The listing builds one solid part. Answer for the finished solid, in the listing's coordinates (mm). Coordinates: 2 decimals unless noted, no trailing zeros. Order: outer loops, then holes, each group sorted by start corner. A loop starts at its lowest first (then second) coordinate and runs counter-clockwise, first axis right, second up. Notation, with made-up numbers: (88.25, 59) -> (113.25, 59) arc R24 ccw to (113.25, 78) -> close; hole circle Ø8 at (78, 10.25). An arc over 180 degrees is marked (long way). Return JSON: item names as keys, results as strings.
```python
from build123d import *

# Parameters (mm, degrees)
BOSS_EXTRUDE1_DEPTH       = 10
FILLET2_R                 = 0.5
SKETCH2_R                 = 1.6
CUT_EXTRUDE1_DEPTH        = 4.896527904
REVISION_INDICATION_DEPTH = 0.4


with BuildPart() as part:
    # Sketch1 → Boss-Extrude1 (new body)
    with BuildSketch(Plane(origin=(0, 0, 0), x_dir=(1, 0, 0), z_dir=(0, 1, 0))):
        Polygon((20.35, 0.1), (14.35, 0.1), (0, 0), (-0.016724739, 2.4), (14.35, 3.9), (20.35, 3.9), (34.716724739, 2.4), (34.7, 0), align=None)
    extrude(amount=BOSS_EXTRUDE1_DEPTH)

    # Fillet2
    fillet2_edges = [part.edges().sort_by_distance(p)[0] for p in [
        (-0.016724739, 5, -2.4),
        (34.716724739, 5, -2.4),
        (34.7, 5, 0),
        (0, 5, 0),
    ]]
    fillet(fillet2_edges, radius=FILLET2_R)

    # Sketch2 → Cut-Extrude1 (cut, through all)
    with BuildSketch(Plane(origin=(0, 0, -3.9), x_dir=(-1, 0, 0), z_dir=(0, 0, -1))):
        with Locations((-17.35, 5)):
            Circle(SKETCH2_R)
    extrude(amount=-CUT_EXTRUDE1_DEPTH, mode=Mode.SUBTRACT)

    # Sketch5 → revision indication (add)
    with BuildSketch(Plane(origin=(-0.248057274, 0, -2.375847049), x_dir=(-0.994593653, 0, 0.103843465), z_dir=(-0.103843465, 0, -0.994593653))):
        with BuildLine():
            add(Edge.make_bspline(
                [(-1.785308798, 1.976923077), (-1.749947985, 1.974821832), (-1.680627244, 1.970702586), (-1.580407683, 1.942442049), (-1.489703086, 1.892261337), (-1.40890887, 1.825381725), (-1.342312834, 1.744291021), (-1.290343795, 1.654309873), (-1.262329436, 1.553251269), (-1.258240196, 1.483528859), (-1.256142132, 1.44775641)],
                knots=[0, 0, 0, 0, 0.000106068, 0.000207934, 0.000309251, 0.000414952, 0.000520654, 0.000622584, 0.00072445, 0.000831784, 0.000831784, 0.000831784, 0.000831784], degree=3))
            add(Edge.make_bspline(
                [(-1.256142132, 1.44775641), (-1.258311293, 1.412843512), (-1.262588847, 1.343995789), (-1.290279579, 1.243699421), (-1.342708899, 1.153662038), (-1.408449529, 1.071471016), (-1.489723058, 1.004449722), (-1.580622123, 0.954695939), (-1.680391977, 0.924411918), (-1.749908735, 0.920554208), (-1.785308798, 0.918589744)],
                knots=[0, 0, 0, 0, 0.000104802, 0.000206668, 0.000308598, 0.000415282, 0.000520984, 0.0006223, 0.000724523, 0.000830591, 0.000830591, 0.000830591, 0.000830591], degree=3))
            add(Edge.make_bspline(
                [(-1.785308798, 0.918589744), (-1.82073437, 0.920483127), (-1.889894366, 0.924179507), (-1.989291812, 0.955317742), (-2.080744455, 1.003983162), (-2.162002161, 1.071595984), (-2.228293388, 1.153239101), (-2.278413725, 1.244319503), (-2.308512996, 1.343708683), (-2.312471536, 1.412786963), (-2.314475465, 1.44775641)],
                knots=[0, 0, 0, 0, 0.000106068, 0.000207073, 0.000309509, 0.000415211, 0.000521895, 0.000623212, 0.000725435, 0.000830237, 0.000830237, 0.000830237, 0.000830237], degree=3))
            add(Edge.make_bspline(
                [(-2.314475465, 1.44775641), (-2.312548513, 1.483587428), (-2.308786377, 1.553543092), (-2.278350536, 1.653690044), (-2.228682266, 1.744709926), (-2.161543907, 1.825258007), (-2.080764113, 1.892726399), (-1.989512426, 1.941829667), (-1.889654975, 1.970931558), (-1.820694086, 1.974891267), (-1.785308798, 1.976923077)],
                knots=[0, 0, 0, 0, 0.000107334, 0.000209557, 0.000310874, 0.000416575, 0.000522277, 0.000624713, 0.000725357, 0.000831425, 0.000831425, 0.000831425, 0.000831425], degree=3))
        make_face()
        with BuildLine():
            add(Edge.make_bspline(
                [(-4.146206234, 1.976923077), (-4.110845421, 1.974821832), (-4.04152468, 1.970702586), (-3.941305118, 1.942442049), (-3.850600522, 1.892261337), (-3.769806306, 1.825381725), (-3.70321027, 1.744291021), (-3.651241231, 1.654309873), (-3.623226872, 1.553251269), (-3.619137632, 1.483528859), (-3.617039568, 1.44775641)],
                knots=[0, 0, 0, 0, 0.000106068, 0.000207934, 0.000309251, 0.000414952, 0.000520654, 0.000622584, 0.00072445, 0.000831784, 0.000831784, 0.000831784, 0.000831784], degree=3))
            add(Edge.make_bspline(
                [(-3.617039568, 1.44775641), (-3.619208729, 1.412843512), (-3.623486283, 1.343995789), (-3.651177015, 1.243699421), (-3.703606335, 1.153662038), (-3.769346965, 1.071471016), (-3.850620494, 1.004449722), (-3.941519559, 0.954695939), (-4.041289413, 0.924411918), (-4.110806171, 0.920554208), (-4.146206234, 0.918589744)],
                knots=[0, 0, 0, 0, 0.000104802, 0.000206668, 0.000308598, 0.000415282, 0.000520984, 0.0006223, 0.000724523, 0.000830591, 0.000830591, 0.000830591, 0.000830591], degree=3))
            add(Edge.make_bspline(
                [(-4.146206234, 0.918589744), (-4.181631806, 0.920483127), (-4.250791802, 0.924179507), (-4.350189248, 0.955317742), (-4.441641891, 1.003983162), (-4.522899597, 1.071595984), (-4.589190824, 1.153239101), (-4.639311161, 1.244319503), (-4.669410431, 1.343708683), (-4.673368972, 1.412786963), (-4.675372901, 1.44775641)],
                knots=[0, 0, 0, 0, 0.000106068, 0.000207073, 0.000309509, 0.000415211, 0.000521895, 0.000623212, 0.000725435, 0.000830237, 0.000830237, 0.000830237, 0.000830237], degree=3))
            add(Edge.make_bspline(
                [(-4.675372901, 1.44775641), (-4.673445949, 1.483587428), (-4.669683813, 1.553543092), (-4.639247972, 1.653690044), (-4.589579702, 1.744709926), (-4.522441343, 1.825258007), (-4.441661549, 1.892726399), (-4.350409862, 1.941829667), (-4.25055241, 1.970931558), (-4.181591522, 1.974891267), (-4.146206234, 1.976923077)],
                knots=[0, 0, 0, 0, 0.000107334, 0.000209557, 0.000310874, 0.000416575, 0.000522277, 0.000624713, 0.000725357, 0.000831425, 0.000831425, 0.000831425, 0.000831425], degree=3))
        make_face()
        with BuildLine():
            add(Edge.make_bspline(
                [(-6.50710367, 1.976923077), (-6.471742857, 1.974821832), (-6.402422116, 1.970702586), (-6.302202554, 1.942442049), (-6.211497957, 1.892261337), (-6.130703742, 1.825381725), (-6.064107706, 1.744291021), (-6.012138667, 1.654309873), (-5.984124308, 1.553251269), (-5.980035068, 1.483528859), (-5.977937003, 1.44775641)],
                knots=[0, 0, 0, 0, 0.000106068, 0.000207934, 0.000309251, 0.000414952, 0.000520654, 0.000622584, 0.00072445, 0.000831784, 0.000831784, 0.000831784, 0.000831784], degree=3))
            add(Edge.make_bspline(
                [(-5.977937003, 1.44775641), (-5.980106165, 1.412843512), (-5.984383719, 1.343995789), (-6.012074451, 1.243699421), (-6.064503771, 1.153662038), (-6.130244401, 1.071471016), (-6.21151793, 1.004449722), (-6.302416994, 0.954695939), (-6.402186849, 0.924411918), (-6.471703607, 0.920554208), (-6.50710367, 0.918589744)],
                knots=[0, 0, 0, 0, 0.000104802, 0.000206668, 0.000308598, 0.000415282, 0.000520984, 0.0006223, 0.000724523, 0.000830591, 0.000830591, 0.000830591, 0.000830591], degree=3))
            add(Edge.make_bspline(
                [(-6.50710367, 0.918589744), (-6.542529242, 0.920483127), (-6.611689237, 0.924179507), (-6.711086684, 0.955317742), (-6.802539327, 1.003983162), (-6.883797033, 1.071595984), (-6.95008826, 1.153239101), (-7.000208597, 1.244319503), (-7.030307867, 1.343708683), (-7.034266408, 1.412786963), (-7.036270337, 1.44775641)],
                knots=[0, 0, 0, 0, 0.000106068, 0.000207073, 0.000309509, 0.000415211, 0.000521895, 0.000623212, 0.000725435, 0.000830237, 0.000830237, 0.000830237, 0.000830237], degree=3))
            add(Edge.make_bspline(
                [(-7.036270337, 1.44775641), (-7.034343385, 1.483587428), (-7.030581249, 1.553543092), (-7.000145408, 1.653690044), (-6.950477138, 1.744709926), (-6.883338779, 1.825258007), (-6.802558985, 1.892726399), (-6.711307298, 1.941829667), (-6.611449846, 1.970931558), (-6.542488958, 1.974891267), (-6.50710367, 1.976923077)],
                knots=[0, 0, 0, 0, 0.000107334, 0.000209557, 0.000310874, 0.000416575, 0.000522277, 0.000624713, 0.000725357, 0.000831425, 0.000831425, 0.000831425, 0.000831425], degree=3))
        make_face()
        with BuildLine():
            add(Edge.make_bspline(
                [(-8.868001106, 1.976923077), (-8.832640293, 1.974821832), (-8.763319552, 1.970702586), (-8.66309999, 1.942442049), (-8.572395393, 1.892261337), (-8.491601178, 1.825381725), (-8.425005142, 1.744291021), (-8.373036103, 1.654309873), (-8.345021744, 1.553251269), (-8.340932504, 1.483528859), (-8.338834439, 1.44775641)],
                knots=[0, 0, 0, 0, 0.000106068, 0.000207934, 0.000309251, 0.000414952, 0.000520654, 0.000622584, 0.00072445, 0.000831784, 0.000831784, 0.000831784, 0.000831784], degree=3))
            add(Edge.make_bspline(
                [(-8.338834439, 1.44775641), (-8.341003601, 1.412843512), (-8.345281155, 1.343995789), (-8.372971887, 1.243699421), (-8.425401207, 1.153662038), (-8.491141837, 1.071471016), (-8.572415366, 1.004449722), (-8.66331443, 0.954695939), (-8.763084284, 0.924411918), (-8.832601042, 0.920554208), (-8.868001106, 0.918589744)],
                knots=[0, 0, 0, 0, 0.000104802, 0.000206668, 0.000308598, 0.000415282, 0.000520984, 0.0006223, 0.000724523, 0.000830591, 0.000830591, 0.000830591, 0.000830591], degree=3))
            add(Edge.make_bspline(
                [(-8.868001106, 0.918589744), (-8.903426678, 0.920483127), (-8.972586673, 0.924179507), (-9.07198412, 0.955317742), (-9.163436763, 1.003983162), (-9.244694469, 1.071595984), (-9.310985696, 1.153239101), (-9.361106033, 1.244319503), (-9.391205303, 1.343708683), (-9.395163844, 1.412786963), (-9.397167773, 1.44775641)],
                knots=[0, 0, 0, 0, 0.000106068, 0.000207073, 0.000309509, 0.000415211, 0.000521895, 0.000623212, 0.000725435, 0.000830237, 0.000830237, 0.000830237, 0.000830237], degree=3))
            add(Edge.make_bspline(
                [(-9.397167773, 1.44775641), (-9.395240821, 1.483587428), (-9.391478685, 1.553543092), (-9.361042844, 1.653690044), (-9.311374574, 1.744709926), (-9.244236214, 1.825258007), (-9.16345642, 1.892726399), (-9.072204734, 1.941829667), (-8.972347282, 1.970931558), (-8.903386394, 1.974891267), (-8.868001106, 1.976923077)],
                knots=[0, 0, 0, 0, 0.000107334, 0.000209557, 0.000310874, 0.000416575, 0.000522277, 0.000624713, 0.000725357, 0.000831425, 0.000831425, 0.000831425, 0.000831425], degree=3))
        make_face()
    extrude(amount=REVISION_INDICATION_DEPTH)


solid = part.part
```
Item 1: The part is cut by section A-A on x = 17.35. Determine the outline of the cut face in (y, z).
Answer list:
{"outline": "(0, -3.9) -> (3.4, -3.9) -> (3.4, -0.1) -> (0, -0.1) -> close; (6.6, -3.9) -> (10, -3.9) -> (10, -0.1) -> (6.6, -0.1) -> close"}
Item 2: Flat-ended cylindrical pins translate along their axes: pin 1 (4 mm diameter, centred on x = 17.35, y = 5, fed in from +Z); pin 2 (1.5 mm diameter, centred on x = 7, y = 9, fed in from -Z); pin 3 (2 mm diameter, centred on x = 11, y = 8, fed in from -Z). Find the tip coordinate at first contact, or state that the pin passes through.
Answer list:
{"pin 1": "z = -0.1", "pin 2": "z = -3.21", "pin 3": "z = -3.65"}
Item 3: The part is cut by section C-C on x = 11.5. Determine the outline of the cut face in (y, z), plus the area to 3 significant figures.
Answer list:
{"outline": "(0, -3.6) -> (10, -3.6) -> (10, -0.08) -> (0, -0.08) -> close", "area": "35.2 mm2"}
Item 4: Find the intervals of material crossed by probe 1 along Y at (x, z) = (17.35, -1.3); probe 2 along Z at (x, y) = (19, 3.75); probe 3 along X at (y, z) = (5.75, -2.3), in increasing order.
Answer list:
{"probe 1": "0 to 3.4, 6.6 to 10", "probe 2": "-3.9 to -0.1", "probe 3": "0.13 to 15.94, 18.76 to 34.57"}
Item 5: The part is cut by section B-B on y = 5. Determine the outline of the cut face in (x, z), plus the area to 3 significant figures.
Answer list:
{"outline": "(-0.01, -1.95) arc R0.5 ccw to (0.43, -2.45) -> (14.35, -3.9) -> (15.75, -3.9) -> (15.75, -0.1) -> (14.35, -0.1) -> (0.5, 0) arc R0.5 ccw to (0, -0.5) -> close; (18.95, -3.9) -> (20.35, -3.9) -> (34.27, -2.45) arc R0.5 ccw to (34.71, -1.95) -> (34.7, -0.5) arc R0.5 ccw to (34.2, 0) -> (20.35, -0.1) -> (18.95, -0.1) -> close", "area": "99.5 mm2"}
Item 6: Determine the mould class of faces 1 (the flat face through (19, 4, -0.1)), 2 (the flat face through (6.17, 1.46, -3.45)), 3 (the flat face through (18, 10, -2)) for opening direction X: pulls with the +X half, pulls with the -X half, needs draft (parallel to the pull), parting line crosses it, or undercut.
Answer list:
{"face 1": "undercut", "face 2": "pulls with the -X half", "face 3": "needs draft"}
